Design review of the part built by this model. Coordinates are the model's own, in mm. Face numbers are marked on the shaded views. A direction names the side the tool comes from. Coordinates: 2 decimals unless noted, no trailing zeros. Write each loop counter-clockwise with the first axis right and the second up, starting at its lowest first coordinate (ties: lowest second). Pieces come first, ordered by that corner, then holes.
Q1. Mouldability with a two-part tool opening along Z and no side actions: class the marked faces 1, 2 and 3 as pulls with the +Z half, pulls with the -Z half, needs draft (parallel to the pull), parting line crosses it, or undercut.
Q2. Insertion check: pin 1 (12 mm diameter, centred on x = 16.5, z = 4, fed in from -Y); pin 2 (8 mm diameter, centred on x = 4.5, y = -3, fed in from -Z); pin 3 (6 mm diameter, centred on y = -11, z = 8, fed in from -X); pin 4 (1.5 mm diameter, centred on x = 5.5, y = 8.5, fed in from -Z). Each pin has a flat end and moves straight along its axis. Give the tip position at first contact, or say it passes through.
Q3. Take a section at B-B (z = -13). Give the boundary of the cut face in (x, y).
Q4. Machinability: for the marked faces 4, 5 and 6, which of the approach directions +Z, -Z, +X, -X, +Y, -Y give a long, thin tool a straight path to every point of the face, cutting with its end or side? Answer none if there is none.
Q5. For probe 1 along Z at (x, y) = (15.5, 0); probe 2 along Y at (x, z) = (9.5, 6); probe 3 along Y at (x, z) = (8.75, 4), list the stretches that pass through material, from the lowest coordinate up.
Q6. Take a section at A-A (x = 12). Give the boundary of the cut face in (y, z), and give its area (3 significant figures).
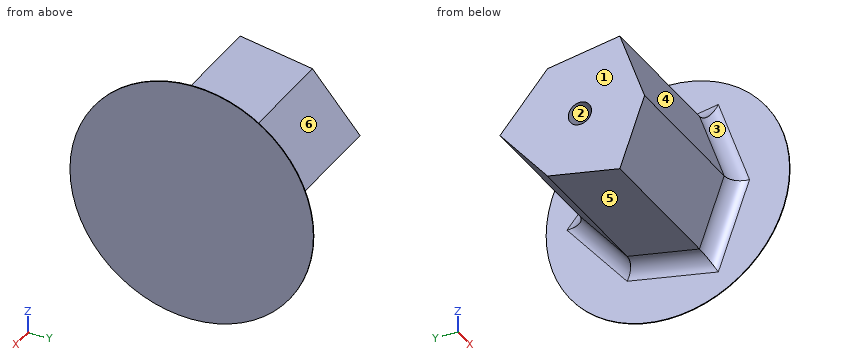
Autodesk Inventor part; units mm, degrees
ref_plane "YZ Plane" through (0, 0, 0) normal (1, 0, 0) x (0, 1, 0)
ref_plane "XZ Plane" through (0, 0, 0) normal (0, 1, 0) x (-1, 0, 0)
ref_plane "XY Plane" through (0, 0, 0) normal (0, 0, 1) x (1, 0, 0)
sketch "Block1" plane through (0, 0, 0) normal (0, 0, 1) x (1, 0, 0)
  line L0 (4.046, 7.0078) -> (10, 0)
  line L1 (4.046, -7.0078) -> (10, 0)
  line L2 (4.046, -7.0078) -> (-5, -8.6603)
  line L3 (-5, -8.6603) -> (-8.092, 0)
  line L4 (-8.092, 0) -> (-5, 8.6603)
  line L5 (-5, 8.6603) -> (4.046, 7.0078)
  point P0 (0, 0)
sketch "Sketch1" plane through (0, 0, 0) normal (1, 0, 0) x (0, 1, 0)
  circle A0 centre (0, 0) radius 1.45
  line L0 (4.046, 7.0078) -> (10, 0)
  line L1 (4.046, -7.0078) -> (10, 0)
  line L2 (4.046, -7.0078) -> (-5, -8.6603)
  line L3 (-5, -8.6603) -> (-8.092, 0)
  line L4 (-8.092, 0) -> (-5, 8.6603)
  line L5 (-5, 8.6603) -> (4.046, 7.0078)
  point P0 (-0.5025, 0)
  point P1 (-0.5025, 0)
  dimension "d3" = 2.9
extrude "Extrusion1" add sketch "Sketch1" along normal blind 21
sketch "Sketch2" plane through (21, 0, 0) normal (1, 0, 0) x (0, 0, -1)
  circle A0 centre (0, 0) radius 15.2315
extrude "Extrusion2" add sketch "Sketch2" along normal blind 0.1
fillet "Fillet1" radius 2 6 edges at (21, 7.023, -3.5039) (21, 7.023, 3.5039) (21, -0.477, 7.834) (21, -6.546, 4.3301) (21, -6.546, -4.3301) (21, -0.477, -7.834)
properties part number "eje motor"
Response:
1. face 1: needs draft
1. face 2: undercut
1. face 3: pulls with the +Z half
2. pin 1: stops at y = -15.23
2. pin 2: stops at z = -8.66
2. pin 3: stops at x = 21
2. pin 4: stops at z = -2.65
3. outline: (21, -7.94) - (21.1, -7.94) - (21.1, 7.94) - (21, 7.94) - close
4. face 4: +Z, -X, -Y
4. face 5: -Z, -X, +Y
4. face 6: +Z, -X, +Y
5. probe 1: z = -7.75 to -1.45, 1.45 to 7.75
5. probe 2: y = -5.95 to 4.9
5. probe 3: y = -6.66 to 6.6
6. outline: (-8.09, 0) - (-5, -8.66) - (4.05, -7.01) - (10, 0) - (4.05, 7.01) - (-5, 8.66) - close; hole circle Ø2.9 at (0, 0)
6. area: 204 mm2
